```python
from build123d import *

# Parameters (mm, degrees)
SKETCH1_R           = 35
BOSS_EXTRUDE1_DEPTH = 26
SKETCH2_R           = 35
SKETCH2_R_2         = 17.5
CUT_EXTRUDE1_DEPTH  = 19
SKETCH3_R           = 2
CUT_EXTRUDE2_DEPTH  = 18
SKETCH4_R           = 5.5
CUT_EXTRUDE4_DEPTH  = 3
CUT_EXTRUDE5_REACH  = 28
SKETCH5_R           = 9.5
SKETCH6_R           = 13
CUT_EXTRUDE6_DEPTH  = 22
CUT_EXTRUDE7_REACH  = 54.5
SKETCH7_R           = 2.5
SKETCH8_R           = 14
CUT_EXTRUDE8_DEPTH  = 8
SKETCH9_R           = 13.6
CUT_EXTRUDE9_DEPTH  = 0.625


with BuildPart() as part:
    # Sketch1 → Boss-Extrude1 (new body)
    with BuildSketch(Plane(origin=(0, 0, 0), x_dir=(0, 0, -1), z_dir=(1, 0, 0))):
        Circle(SKETCH1_R)
    extrude(amount=-BOSS_EXTRUDE1_DEPTH)

    # Sketch2 → Cut-Extrude1 (cut)
    with BuildSketch(Plane.ZY.offset(26)):
        Circle(SKETCH2_R)
        Circle(SKETCH2_R_2, mode=Mode.SUBTRACT)
    extrude(amount=-CUT_EXTRUDE1_DEPTH, mode=Mode.SUBTRACT)

    # Sketch3 → Cut-Extrude2 (cut)
    with BuildSketch(Plane.ZY.offset(7)):
        with Locations((0, 28.33)):
            Circle(SKETCH3_R)
        with Locations((28.33, 0)):
            Circle(SKETCH3_R)
        with Locations((0, -28.33)):
            Circle(SKETCH3_R)
        with Locations((-28.33, 0)):
            Circle(SKETCH3_R)
    extrude(amount=-CUT_EXTRUDE2_DEPTH, mode=Mode.SUBTRACT)

    # Sketch4 → Cut-Extrude4 (cut)
    with BuildSketch(Plane.ZY.offset(7)):
        with Locations((0, 28.33)):
            Circle(SKETCH4_R)
        with Locations((28.33, 0)):
            Circle(SKETCH4_R)
        with Locations((0, -28.33)):
            Circle(SKETCH4_R)
        with Locations((-28.33, 0)):
            Circle(SKETCH4_R)
    extrude(amount=-CUT_EXTRUDE4_DEPTH, mode=Mode.SUBTRACT)

    # Sketch5 → Cut-Extrude5 (cut, up to next)
    with BuildSketch(Plane.ZY.offset(26), mode=Mode.PRIVATE) as cut_extrude5_sk1:
        Circle(SKETCH5_R)
    cut_extrude5_tool1 = extrude(cut_extrude5_sk1.sketch, amount=-CUT_EXTRUDE5_REACH, mode=Mode.PRIVATE) & part.part
    add(cut_extrude5_tool1.solids().sort_by_distance((-26, 0, 0))[0], mode=Mode.SUBTRACT)

    # Sketch6 → Cut-Extrude6 (cut)
    with BuildSketch(Plane(origin=(0, 0, 0), x_dir=(0, 0, -1), z_dir=(1, 0, 0))):
        Circle(SKETCH6_R)
    extrude(amount=-CUT_EXTRUDE6_DEPTH, mode=Mode.SUBTRACT)

    # Sketch7 → Cut-Extrude7 (cut, up to next)
    with BuildSketch(Plane(origin=(0, 17.5, 0), x_dir=(1, 0, 0), z_dir=(0, 1, 0)), mode=Mode.PRIVATE) as cut_extrude7_sk1:
        with Locations((-11, 0)):
            Circle(SKETCH7_R)
    cut_extrude7_tool1 = extrude(cut_extrude7_sk1.sketch, amount=-CUT_EXTRUDE7_REACH, mode=Mode.PRIVATE) & part.part
    add(cut_extrude7_tool1.solids().sort_by_distance((-11, 17.5, 0))[0], mode=Mode.SUBTRACT)

    # Sketch8 → Cut-Extrude8 (cut)
    with BuildSketch(Plane(origin=(0, 0, 0), x_dir=(0, 0, -1), z_dir=(1, 0, 0))):
        Circle(SKETCH8_R)
    extrude(amount=-CUT_EXTRUDE8_DEPTH, mode=Mode.SUBTRACT)

    # Sketch9 → Cut-Extrude9 (cut, symmetric)
    with BuildSketch(Plane(origin=(-16.35, 0, 0), x_dir=(0, 0, -1), z_dir=(1, 0, 0))):
        Circle(SKETCH9_R)
    extrude(amount=CUT_EXTRUDE9_DEPTH, both=True, mode=Mode.SUBTRACT)


solid = part.part
```
Build history of the part. All positions in model axes, mm. A direction names the side the tool comes from. Round coordinates to 2 decimals unless told otherwise and drop trailing zeros. Write each loop counter-clockwise with the first axis right and the second up, starting at its lowest first coordinate (ties: lowest second). Pieces come first, ordered by that corner, then holes. Notation, with made-up numbers: (-35.5, -32.5) - (-22.5, -32.5) arc R23 ccw to (-22.5, -7.5) - close; hole circle Ø8 at (51.5, -8.5). An arc over 180 degrees is marked (long way). Write each question's results on one line, items separated by ' | '. Start each with the question number.
Item 1: Saw through at D-D (z = 10.5). Write the cut outline in (x, y) (1 decimal).
Item 2: Mould opens along Z. For faces 1 (the face through (-2.028, 0.088, 26.332)), 2 (the face through (-7, 8, -16)), 3 (the face through (-16.633, -17.084, -3.794)), 4 (the face through (-5.52, 22.96, -1.19)) say: pulls with the +Z half, pulls with the -Z half, needs draft (parallel to the pull), parting line crosses it, or undercut.
Item 3: Drop flat-ended pins along their axis: P1, Ø3.5, axis at y = -1, z = -31, coming from the -X side; P2, Ø1, axis at x = -2.5, z = -17, coming from the -Y side; P3, Ø8, axis at x = -6, z = 27.5, coming from the +Y side. Give the stop position or say it passes through.
Item 4: Saw through at C-C (x = -20.75). Write the cut outline in (y, z), and give its area (3 significant figures).
Item 5: Saw through at A-A (y = -28.33). Write the cut outline in (x, z), and give its area (3 significant figures).
Item 6: Which spindle directions (+Z, -Z, +X, -X, +Y, -Y) get a long thin tool onto all of the face, cutting with end or side? Do faces 5 (the face through (-26, -8, -8)), 6 (the face through (-3.944, -5.362, -12.932)), 7 (the face through (-4, -31, 0)), 8 (the face through (-3, -21, 28)), 9 (the face through (-16.341, -13.277, 2.948)). Say none if no direction does.
Item 7: Wall check: L1, parallel to Y at x = -5, z = 5; L2, parallel to Y at x = -16.4, z = 0; L3, parallel to Y at x = -2.75, z = -17.5. Give the ranges that are in metal, low to high. Write a range as [from, to].
Results are:
1) outline: (-26, -14) - (-7, -14) - (-7, -33.4) - (0, -33.4) - (0, -9.3) - (-8, -9.3) - (-8, -7.7) - (-15.7, -7.7) - (-15.7, -8.6) - (-17, -8.6) - (-17, -7.7) - (-22, -7.7) - (-22, 7.7) - (-17, 7.7) - (-17, 8.6) - (-15.7, 8.6) - (-15.7, 7.7) - (-8, 7.7) - (-8, 9.3) - (0, 9.3) - (0, 33.4) - (-7, 33.4) - (-7, 14) - (-26, 14) - close
2) face 1: undercut | face 2: needs draft | face 3: parting line crosses it | face 4: undercut
3) P1: stops at x = -4 | P2: stops at y = -30.87 | P3: stops at y = 25.94
4) outline: circle Ø35 at (0, 0); hole circle Ø26 at (0, 0) | area: 431 mm²
5) outline: (-7, -20.55) - (0, -20.55) - (0, -2) - (-4, -2) - (-4, -5.5) - (-7, -5.5) - close; (-7, 5.5) - (-4, 5.5) - (-4, 2) - (0, 2) - (0, 20.55) - (-7, 20.55) - close | area: 239 mm²
6) face 5: +Z, -Z, -X, +Y, -Y | face 6: +X | face 7: -X | face 8: +X, -X | face 9: none
7) L1: y = [-34.64, -30.62], [-26.04, -13.08], [13.08, 26.04], [30.62, 34.64] | L2: y = [-17.5, -13.6], [13.6, 17.5] | L3: y = [-30.31, 30.31]
